Can you work these out from the model? Positions are in its coordinate system, mm. Face numbers are marked on the shaded views. A direction names the side the tool comes from. Give positions to 0.01 mm unless a question says otherwise; leave off trailing zeros. Write each loop counter-clockwise with the first axis right and the second up, starting at its lowest first coordinate (ties: lowest second). Pieces come first, ordered by that corner, then holes. Notation, with made-up numbers: (-21.5, 8.25) - (0.5, 8.25) arc R31 cw to (0.5, 36.25) - close; hole circle Ø1 at (30.25, 79.5). An arc over 180 degrees is marked (long way). Return JSON: item names as keys, results as strings. Group by question number.
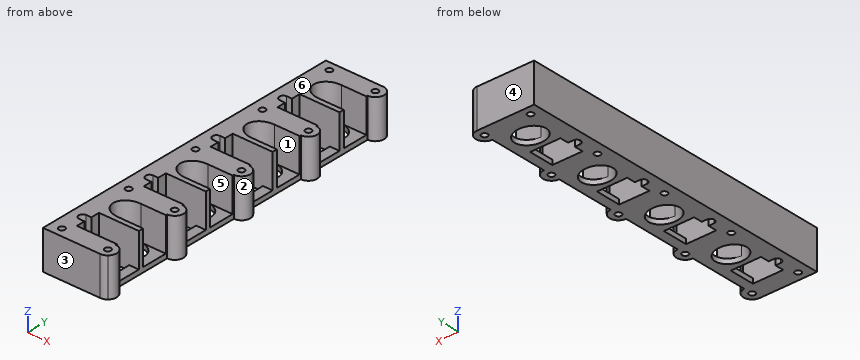
from build123d import *

# Parameters (mm, degrees)
F0_R     = 4
F1_DEPTH = 50.8
F3_W     = 32.512
F3_H     = 33.750834
F3_H_2   = 33.02
F4_DEPTH = 44.45


with BuildPart() as f1:
    # F0 (on Top) → F1 (new body)
    with BuildSketch(Plane.XY):
        with BuildLine():
            ThreePointArc((-7.62, 399.288), (3.8735, 410.7815), (-7.62, 422.275))
            Line((-7.62, 422.275), (-82.55, 422.275))
            Line((-82.55, 422.275), (-82.55, 0))
            Line((-82.55, 0), (-7.62, 0))
            ThreePointArc((-7.62, 0), (-3.545348, 0.746512), (0, 2.889074))
            ThreePointArc((0, 2.889074), (3.126988, 15.568152), (-7.62, 22.987))
            Line((-7.62, 22.987), (-7.62, 99.822))
            ThreePointArc((-7.62, 99.822), (3.8735, 111.3155), (-7.62, 122.809))
            Line((-7.62, 122.809), (-7.62, 199.644))
            ThreePointArc((-7.62, 199.644), (3.8735, 211.1375), (-7.62, 222.631))
            Line((-7.62, 222.631), (-7.62, 299.466))
            ThreePointArc((-7.62, 299.466), (3.8735, 310.9595), (-7.62, 322.453))
            Line((-7.62, 322.453), (-7.62, 399.288))
        make_face()
        with Locations((-67.945, 11.4935)):
            Circle(F0_R, mode=Mode.SUBTRACT)
        with BuildLine():
            Line((-59.944, 57.8485), (-20.32, 57.8485))
            Line((-20.32, 57.8485), (-20.32, 24.8285))
            Line((-20.32, 24.8285), (-59.944, 24.8285))
            Line((-59.944, 24.8285), (-59.944, 36.2585))
            Line((-59.944, 36.2585), (-66.802, 36.2585))
            ThreePointArc((-66.802, 36.2585), (-71.882, 41.3385), (-66.802, 46.4185))
            Line((-66.802, 46.4185), (-59.944, 46.4185))
            Line((-59.944, 46.4185), (-59.944, 57.8485))
        make_face(mode=Mode.SUBTRACT)
        with BuildLine():
            add(Edge.make_bspline(
                [(-20.32, 81.0895), (-20.32, 110.34557), (-51.3715, 95.717535), (-82.423, 81.0895), (-51.3715, 66.461465), (-20.32, 51.83343), (-20.32, 81.0895)],
                knots=[0, 0, 0, 2.094395, 2.094395, 4.18879, 4.18879, 6.283185, 6.283185, 6.283185], degree=2, weights=[1, 0.5, 1, 0.5, 1, 0.5, 1]))
        make_face(mode=Mode.SUBTRACT)
        with Locations((-67.945, 111.3155)):
            Circle(F0_R, mode=Mode.SUBTRACT)
        with BuildLine():
            Line((-59.944, 157.6705), (-20.32, 157.6705))
            Line((-20.32, 157.6705), (-20.32, 124.6505))
            Line((-20.32, 124.6505), (-59.944, 124.6505))
            Line((-59.944, 124.6505), (-59.944, 136.0805))
            Line((-59.944, 136.0805), (-66.802, 136.0805))
            ThreePointArc((-66.802, 136.0805), (-71.882, 141.1605), (-66.802, 146.2405))
            Line((-66.802, 146.2405), (-59.944, 146.2405))
            Line((-59.944, 146.2405), (-59.944, 157.6705))
        make_face(mode=Mode.SUBTRACT)
        with BuildLine():
            add(Edge.make_bspline(
                [(-20.32, 180.9115), (-20.32, 210.16757), (-51.3715, 195.539535), (-82.423, 180.9115), (-51.3715, 166.283465), (-20.32, 151.65543), (-20.32, 180.9115)],
                knots=[0, 0, 0, 2.094395, 2.094395, 4.18879, 4.18879, 6.283185, 6.283185, 6.283185], degree=2, weights=[1, 0.5, 1, 0.5, 1, 0.5, 1]))
        make_face(mode=Mode.SUBTRACT)
        with Locations((-7.62, 11.4935)):
            Circle(F0_R, mode=Mode.SUBTRACT)
        with Locations((-7.62, 111.3155)):
            Circle(F0_R, mode=Mode.SUBTRACT)
        with Locations((-67.945, 211.1375)):
            Circle(F0_R, mode=Mode.SUBTRACT)
        with Locations((-67.945, 310.9595)):
            Circle(F0_R, mode=Mode.SUBTRACT)
        with BuildLine():
            Line((-59.944, 257.4925), (-20.32, 257.4925))
            Line((-20.32, 257.4925), (-20.32, 224.4725))
            Line((-20.32, 224.4725), (-59.944, 224.4725))
            Line((-59.944, 224.4725), (-59.944, 235.9025))
            Line((-59.944, 235.9025), (-66.802, 235.9025))
            ThreePointArc((-66.802, 235.9025), (-71.882, 240.9825), (-66.802, 246.0625))
            Line((-66.802, 246.0625), (-59.944, 246.0625))
            Line((-59.944, 246.0625), (-59.944, 257.4925))
        make_face(mode=Mode.SUBTRACT)
        with BuildLine():
            add(Edge.make_bspline(
                [(-20.32, 280.7335), (-20.32, 309.98957), (-51.3715, 295.361535), (-82.423, 280.7335), (-51.3715, 266.105465), (-20.32, 251.47743), (-20.32, 280.7335)],
                knots=[0, 0, 0, 2.094395, 2.094395, 4.18879, 4.18879, 6.283185, 6.283185, 6.283185], degree=2, weights=[1, 0.5, 1, 0.5, 1, 0.5, 1]))
        make_face(mode=Mode.SUBTRACT)
        with Locations((-67.945, 410.7815)):
            Circle(F0_R, mode=Mode.SUBTRACT)
        with BuildLine():
            Line((-59.944, 357.3145), (-20.32, 357.3145))
            Line((-20.32, 357.3145), (-20.32, 324.2945))
            Line((-20.32, 324.2945), (-59.944, 324.2945))
            Line((-59.944, 324.2945), (-59.944, 335.7245))
            Line((-59.944, 335.7245), (-66.802, 335.7245))
            ThreePointArc((-66.802, 335.7245), (-71.882, 340.8045), (-66.802, 345.8845))
            Line((-66.802, 345.8845), (-59.944, 345.8845))
            Line((-59.944, 345.8845), (-59.944, 357.3145))
        make_face(mode=Mode.SUBTRACT)
        with BuildLine():
            add(Edge.make_bspline(
                [(-20.32, 380.5555), (-20.32, 409.81157), (-51.3715, 395.183535), (-82.423, 380.5555), (-51.3715, 365.927465), (-20.32, 351.29943), (-20.32, 380.5555)],
                knots=[0, 0, 0, 2.094395, 2.094395, 4.18879, 4.18879, 6.283185, 6.283185, 6.283185], degree=2, weights=[1, 0.5, 1, 0.5, 1, 0.5, 1]))
        make_face(mode=Mode.SUBTRACT)
        with Locations((-7.62, 211.1375)):
            Circle(F0_R, mode=Mode.SUBTRACT)
        with Locations((-7.62, 310.9595)):
            Circle(F0_R, mode=Mode.SUBTRACT)
        with Locations((-7.62, 410.7815)):
            Circle(F0_R, mode=Mode.SUBTRACT)
    extrude(amount=F1_DEPTH)

    # F3 (on face) → F4 (cut)
    with BuildSketch(Plane.XY.offset(50.8)):
        with Locations((-23.876, 81.0895)):
            Rectangle(F3_W, F3_H)
        with Locations((-23.876, 41.3385)):
            Rectangle(F3_W, F3_H_2)
        with Locations((-23.876, 141.1605)):
            Rectangle(F3_W, F3_H_2)
        with Locations((-23.876, 180.9115)):
            Rectangle(F3_W, F3_H)
        with Locations((-23.876, 240.9825)):
            Rectangle(F3_W, F3_H_2)
        with Locations((-23.876, 280.7335)):
            Rectangle(F3_W, F3_H)
        with Locations((-23.876, 340.8045)):
            Rectangle(F3_W, F3_H_2)
        with Locations((-23.876, 380.5555)):
            Rectangle(F3_W, F3_H)
    extrude(amount=-F4_DEPTH, mode=Mode.SUBTRACT)


solid = f1.part
1) I need wall thicknesses on line 1 along X through (y, z) = (314.5, 29); line 2 along X through (y, z) = (280, 41.5); line 3 along X through (y, z) = (124, 5.5). Which ranges of each line are inside material? Lowest first, please.
2) We'd pull the mould along Y, two halves only. Please class the marked faces 3, 4, 5 and 6: pulls with the +Y half, pulls with the -Y half, needs draft (parallel to the pull), parting line crosses it, or undercut.
3) Will these pins go through, and if not, where does the flat tip stop? pin 1 Ø9 at (y, z) = (152.5, 23.5) entering from +X; pin 2 Ø1.5 at (x, y) = (-57.5, 251.5) entering from +Z; pin 3 Ø10 at (x, y) = (-16.5, 46.5) entering from +Z.
4) Imagine slicing it at B-B, the plane x = -32.5. Count the separate pieces of the cut face and the enclosed holes in it, and give its area (3 significant figures).
5) Imagine slicing it at A-A, the plane y = 253. Write out the boundary of the cut face in (x, z).
6) On a 3-axis mill with a long thin cutter (end or side, diameter ignored), from which of +Z, -Z, +X, -X, +Y, -Y can I reach the whole of each face in a straight line? I mean the marked faces 1 and 2. Say none if no direction works.
Resolved:
{
 "1": {"line 1": "-82.55 to -69.81, -66.08 to -9.48, -5.76 to 3.31", "line 2": "-82.55 to -61.7", "line 3": "-82.55 to -7.62"},
 "2": {"face 3": "pulls with the -Y half", "face 4": "pulls with the +Y half", "face 5": "undercut", "face 6": "needs draft"},
 "3": {"pin 1": "x = -59.94", "pin 2": "through", "pin 3": "z = 6.35"},
 "4": {"separate pieces": "9", "enclosed holes": "0", "area": "7,960 mm^2"},
 "5": {"outline": "(-82.55, 0) - (-59.94, 0) - (-59.94, 50.8) - (-82.55, 50.8) - close; (-20.32, 0) - (-7.62, 0) - (-7.62, 6.35) - (-20.32, 6.35) - close"},
 "6": {"face 1": "+Z, +X", "face 2": "+Z, -Z, +X"}
}
